The figure shows three views and two pictorial views of one solid part (mm, origin at its lowest corner). Answer the questions. A direction names the side the tool comes from. Coordinates: 2 decimals unless noted, no trailing zeros. Write each loop counter-clockwise with the first axis right and the second up, starting at its lowest first coordinate (ties: lowest second). Pieces come first, ordered by that corner, then holes.
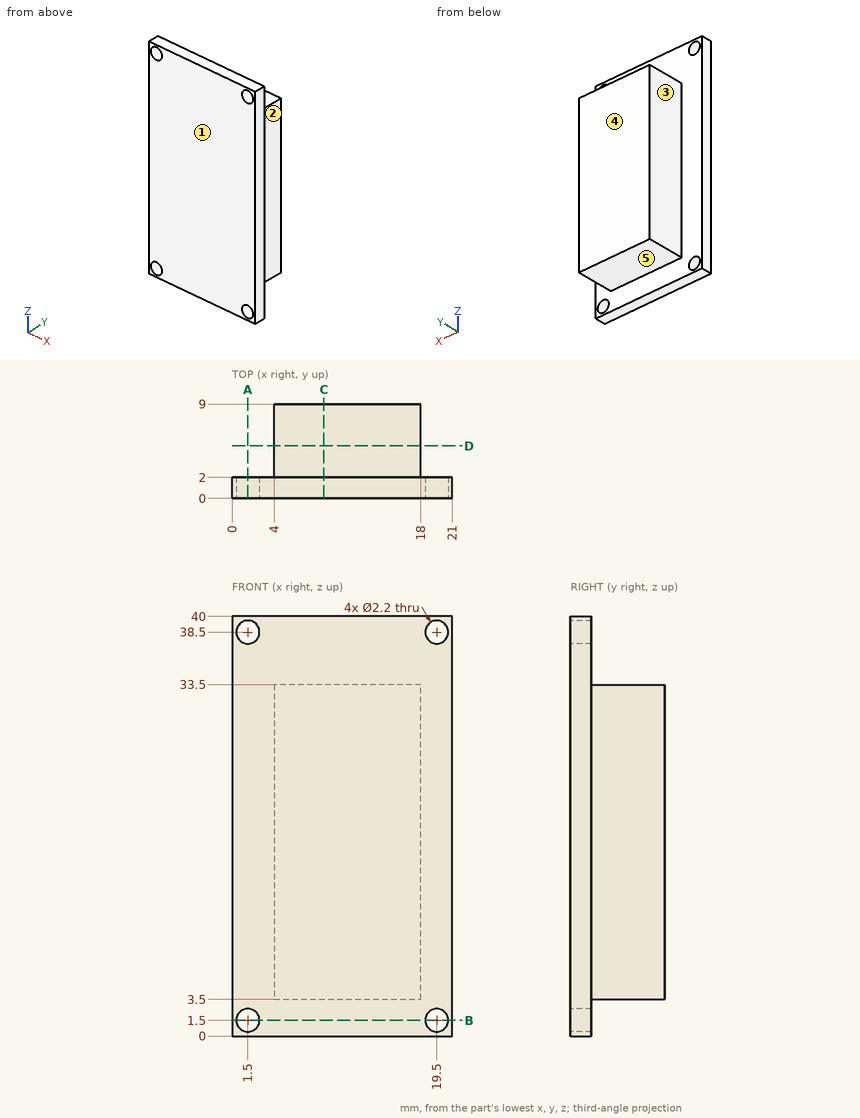
1. Section B-B on z = 1.5 is taken. Give the vertices of the cut face in (x, y), then the cut area to 3 significant figures.
Results found:
outline: (0, 0) - (0.4, 0) - (0.4, 2) - (0, 2) - close; (2.6, 0) - (18.4, 0) - (18.4, 2) - (2.6, 2) - close; (20.6, 0) - (21, 0) - (21, 2) - (20.6, 2) - close
area: 33.2 mm2
2. For a pull along Z with two mould halves and no side action, classify the marked faces 4 and 5 as pulls with the +Z half, pulls with the -Z half, needs draft (parallel to the pull), parting line crosses it, or undercut.
Results found:
face 4: needs draft
face 5: pulls with the -Z half
3. Section D-D on y = 5 is taken. Give the vertices of the cut face in (x, z), then the cut area to 3 significant figures.
Results found:
outline: (4, 3.5) - (18, 3.5) - (18, 33.5) - (4, 33.5) - close
area: 420 mm2
4. Section C-C on x = 8.75 is taken. Give the vertices of the cut face in (y, z), then the cut area to 3 significant figures.
Results found:
outline: (0, 0) - (2, 0) - (2, 3.5) - (9, 3.5) - (9, 33.5) - (2, 33.5) - (2, 40) - (0, 40) - close
area: 290 mm2
5. A tool of negligible diameter and unlimited length cuts with its end or side. For the marked faces 1, 2 and 3, from which of +Z, -Z, +X, -X, +Y, -Y can it reach the whole face along a straight path? Write none if from no direction.
Results found:
face 1: +Z, -Z, +X, -X, -Y
face 2: +Z, -Z, +X, +Y
face 3: +Z, -Z, -X, +Y
6. Find the intervals of material crossed by L1, parallel to Z at x = 1.5, y = 0.7; L2, parallel to X at y = 1.45, z = 1.5; L3, parallel to X at y = 2.5, z = 20.5, in increasing order.
Results found:
L1: z = 0 to 0.4, 2.6 to 37.4, 39.6 to 40
L2: x = 0 to 0.4, 2.6 to 18.4, 20.6 to 21
L3: x = 4 to 18
7. Flat-ended cylindrical pins translate along their axes: P1, Ø3.5, axis at x = 19.5, z = 38.5, coming from the +Y side; P2, Ø1.3, axis at x = 19.5, z = 1.5, coming from the +Y side; P3, Ø1, axis at x = 5.5, y = 7.5, coming from the -Z side; P4, Ø2, axis at y = 5, z = 21.5, coming from the +X side. Find the tip coordinate at first contact, or state that the pin passes through.
Results found:
P1: stops at y = 2
P2: passes through
P3: stops at z = 3.5
P4: stops at x = 18
8. Section A-A on x = 1.5 is taken. Give the vertices of the cut face in (y, z), then the cut area to 3 significant figures.
Results found:
outline: (0, 0) - (2, 0) - (2, 0.4) - (0, 0.4) - close; (0, 2.6) - (2, 2.6) - (2, 37.4) - (0, 37.4) - close; (0, 39.6) - (2, 39.6) - (2, 40) - (0, 40) - close
area: 71.2 mm2
